```python
from build123d import *

# Parameters (mm, degrees)
BOSS_EXTRUDE1_DEPTH      = 10
BOSS_EXTRUDE1_DEPTH_BACK = 10
BOSS_EXTRUDE2_DEPTH      = 25
BOSS_EXTRUDE2_DEPTH_BACK = 25
SKETCH2_W                = 10
SKETCH2_H                = 7.5


with BuildPart() as part:
    # Sketch1 → Boss-Extrude1 (new, two sides: drawn at the far end of the back side and taken through both)
    with BuildSketch(Plane(origin=(0, 0, 0), x_dir=(1, 0, 0), z_dir=(0, 1, 0)).offset(-BOSS_EXTRUDE1_DEPTH_BACK)):
        with BuildLine():
            Line((1.407e-06, -32.5), (1.407e-06, -40))
            ThreePointArc((1.407e-06, -40), (15.307339245, -36.955180493), (28.284273238, -28.284269257))
            Line((28.284273238, -28.284269257), (22.980972379, -22.980968398))
            ThreePointArc((22.980972379, -22.980968398), (12.437213502, -30.026083999), (1.407e-06, -32.5))
        make_face()
        with BuildLine():
            ThreePointArc((-22.980970389, -22.980970389), (-12.437210902, -30.026085076), (1.407e-06, -32.5))
            Line((1.407e-06, -32.5), (1.407e-06, -40))
            ThreePointArc((1.407e-06, -40), (-15.307336644, -36.95518157), (-28.284271247, -28.284271247))
            Line((-28.284271247, -28.284271247), (-22.980970389, -22.980970389))
        make_face()
    extrude(amount=BOSS_EXTRUDE1_DEPTH + BOSS_EXTRUDE1_DEPTH_BACK)

    # Sketch2 → Boss-Extrude2 (add, two sides: drawn at the far end of the back side and taken through both)
    with BuildSketch(Plane(origin=(0, 0, 0), x_dir=(1, 0, 0), z_dir=(0, 1, 0)).offset(-BOSS_EXTRUDE2_DEPTH_BACK)):
        Polygon((1.328609333, -41.5), (1.328609333, -45), (5, -45), (5, -40), (-5, -40), (-5, -45), (-1.328609333, -45), (-1.328609333, -41.5), align=None)
        with Locations((0, -36.25)):
            Rectangle(SKETCH2_W, SKETCH2_H)
        with BuildLine():
            Line((0, -32.5), (5, -32.5))
            Line((5, -32.5), (5, -32.113081447))
            ThreePointArc((5, -32.113081447), (2.507474126, -32.403125984), (0, -32.5))
        make_face()
        with BuildLine():
            Line((-5, -32.113081447), (-5, -32.5))
            Line((-5, -32.5), (0, -32.5))
            ThreePointArc((0, -32.5), (-2.507474126, -32.403125984), (-5, -32.113081447))
        make_face()
    extrude(amount=BOSS_EXTRUDE2_DEPTH + BOSS_EXTRUDE2_DEPTH_BACK)


solid = part.part
```
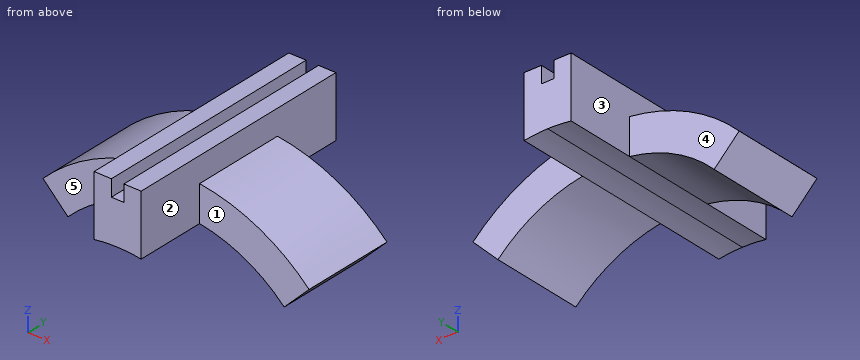
Geometry check sheet. Reference: the model listing, model coordinates, mm. Face numbers are marked on the shaded views. A direction names the side the tool comes from. Coordinates: 2 decimals unless noted, no trailing zeros. Order: outer loops, then holes, each group sorted by start corner. A loop starts at its lowest first (then second) coordinate and runs counter-clockwise, first axis right, second up. Notation, with made-up numbers: (51, -38) - (81, -38) arc R36 cw to (81, -3) - close; hole circle Ø9 at (34.5, 3). An arc over 180 degrees is marked (long way). Answer as a JSON object with one key per item and string values. Group by question number.
Item 1: Sectioned sample at B-B, the plane z = 30. Record the cut outline in (x, y).
Item 2: Sectioned sample at A-A, the plane y = 8. Record the cut outline in (x, z), and give its area (3 significant figures).
Item 3: Sectioned sample at D-D, the plane y = -19. Record the cut outline in (x, z).
Item 4: Depth check by flat-ended pin: pin 1 Ø2 at (x, y) = (-16.5, -10) entering from +Z; pin 2 Ø1.8 at (y, z) = (-7, 43.5) entering from -X; pin 3 Ø5 at (x, z) = (-20.5, 35) entering from +Y. Enter the tip coordinate at first touch or a pass-through.
Item 5: Sectioned sample at C-C, the plane z = 38. Record the cut outline in (x, y).
Item 6: Tool access check on the marked faces 1, 2, 3, 4 and 5. Record the directions out of +Z, -Z, +X, -X, +Y, -Y that give a thin tool (end or side, any length) a straight path to the whole face; none if there is none.
Item 7: Scan lines: probe 1 along X at (y, z) = (-7, 43); probe 2 along X at (y, z) = (-20.5, 40.5); probe 3 along Y at (x, z) = (-16, 33). Record each from-to range of solid material in increasing order.
Resolved:
{
 "1": {"outline": "(-26.46, -10) - (-12.5, -10) - (-12.5, 10) - (-26.46, 10) - close; (12.5, -10) - (26.46, -10) - (26.46, 10) - (12.5, 10) - close"},
 "2": {"outline": "(-28.28, 28.28) - (-22.98, 22.98) arc R32.5 cw to (22.98, 22.98) - (28.28, 28.28) arc R40 ccw to (5, 39.69) - (5, 45) - (1.33, 45) - (1.33, 41.5) - (-1.33, 41.5) - (-1.33, 45) - (-5, 45) - (-5, 39.69) arc R40 ccw to start", "area": "469 mm^2"},
 "3": {"outline": "(-5, 32.11) arc R32.5 cw to (5, 32.11) - (5, 45) - (1.33, 45) - (1.33, 41.5) - (-1.33, 41.5) - (-1.33, 45) - (-5, 45) - close"},
 "4": {"pin 1": "z = 36.87", "pin 2": "x = -5", "pin 3": "y = 10"},
 "5": {"outline": "(-12.49, -10) - (-5, -10) - (-5, -25) - (5, -25) - (5, -10) - (12.49, -10) - (12.49, 10) - (5, 10) - (5, 25) - (-5, 25) - (-5, 10) - (-12.49, 10) - close"},
 "6": {"face 1": "+Z, -Z, +X, -Y", "face 2": "+Z, +X", "face 3": "+Z, -X", "face 4": "+Z, -Z, -X, +Y", "face 5": "+Z, -Z, -X, -Y"},
 "7": {"probe 1": "-5 to -1.33, 1.33 to 5", "probe 2": "-5 to 5", "probe 3": "-10 to 10"}
}
